Study the drawing (mm; zero at the part's minimum x, y, z) and answer. A direction names the side the tool comes from. Give positions to 0.01 mm unless a question says otherwise; leave off trailing zeros. Loops run counter-clockwise (first coordinate to the right, second up) from the corner with the lowest first, then second, coordinate; pieces in that order, holes last. Notation, with made-up numbers: M -1,56 L 30,56 A11 cw 30,70 Z; hole C 70.5,20.25 d4. An arc over 180 degrees is marked long. Use one line per item in the form item = value. Start each with the question number.
1. For the marked faces 1, 2 and 3, determine the directions among +Z, -Z, +X, -X, +Y, -Y from which every point of the face is accessible in a straight line to the end or side of a thin tool.
2. Each of these flat-tipped pins is pushed along its axis until it touches: pin 1 Ø10 at (y, z) = (125, 38.5) entering from -X; pin 2 Ø1 at (y, z) = (143, 32.5) entering from +X; pin 3 Ø8 at (x, z) = (152.5, 49) entering from +Y. Where does it stop, or does it pass through?
3. Straight lines are drawn through the part: line 1 (Y direction, x = 20, z = 3.75); line 2 (Z direction, x = 151, y = 87); line 3 (Z direction, x = 244.5, y = 58.5). For each, find the intervals that lie inside material, in ascending order. Write a range as from..to.
4. The part is cut by section B-B (y = 13.5). Write down the section's boundary in (x, z), and give its area (3 significant figures).
5. The part is cut by section C-C (z = 27). Write down the section's boundary in (x, y).
6. The part is cut by section D-D (x = 239.5). Write down the section's boundary in (y, z).
7. The part is cut by section A-A (y = 87.5). Write down the section's boundary in (x, z), and give its area (3 significant figures).
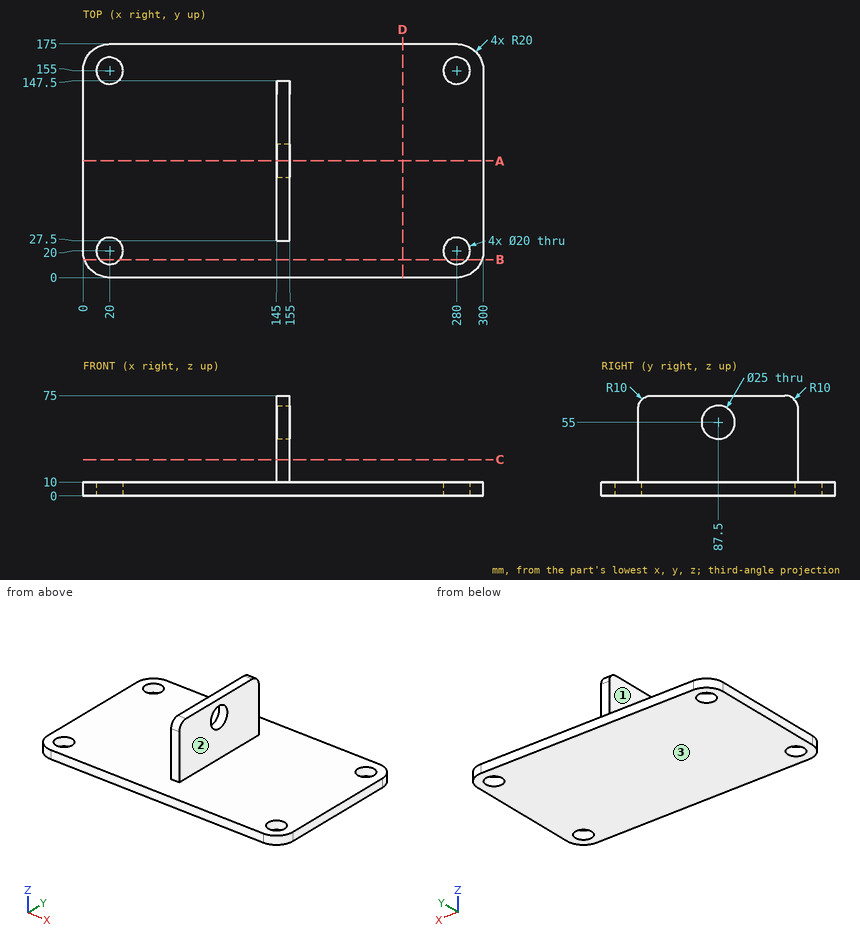
Derived:
q1.face_1 = +Z, -X, +Y, -Y
q1.face_2 = +Z, +X, +Y, -Y
q1.face_3 = -Z, +X, -X, +Y, -Y
q2.pin_1 = 145
q2.pin_2 = 155
q2.pin_3 = 147.5
q3.line_1 = 0..10, 30..145, 165..175
q3.line_2 = 0..42.51, 67.49..75
q3.line_3 = 0..10
q4.outline = M 1.09,0 L 12.4,0 L 12.4,10 L 1.09,10 Z; M 27.6,0 L 272.4,0 L 272.4,10 L 27.6,10 Z; M 287.6,0 L 298.91,0 L 298.91,10 L 287.6,10 Z
q4.area = 2,670 mm2
q5.outline = M 145,27.5 L 155,27.5 L 155,147.5 L 145,147.5 Z
q6.outline = M 0,0 L 175,0 L 175,10 L 0,10 Z
q7.outline = M 0,0 L 300,0 L 300,10 L 155,10 L 155,42.5 L 145,42.5 L 145,10 L 0,10 Z; M 145,67.5 L 155,67.5 L 155,75 L 145,75 Z
q7.area = 3,400 mm2
